from build123d import *

# Parameters (mm, degrees)
BOSS_EXTRUDE1_DEPTH = 12
SKETCH2_R           = 2.5
CUT_EXTRUDE2_DEPTH  = 1.6
SKETCH3_R           = 3
CUT_EXTRUDE3_DEPTH  = 1.6
FILLET2_R           = 1
FILLET3_R           = 1
FILLET4_R           = 1
FILLET5_R           = 1
FILLET6_R           = 1
FILLET7_R           = 1
FILLET8_R           = 1
FILLET9_R           = 1


with BuildPart() as part:
    # Sketch1 → Boss-Extrude1 (new body)
    with BuildSketch(Plane.XY):
        Polygon((-22.976789636, 1.251050745), (-7.976789636, 1.251050745), (-7.976789636, 15.251050745), (7.976789636, 15.251050745), (7.976789636, 1.251050745), (22.976789636, 1.251050745), (22.976789636, -0.348949255), (6.376789636, -0.348949255), (6.376789636, 13.651050745), (-6.376789636, 13.651050745), (-6.376789636, -0.348949255), (-22.976789636, -0.348949255), align=None)
    extrude(amount=BOSS_EXTRUDE1_DEPTH)

    # Sketch2 → Cut-Extrude2 (cut)
    with BuildSketch(Plane(origin=(0, 1.251050745, 0), x_dir=(1, 0, 0), z_dir=(0, 1, 0))):
        with Locations(Location((-16.976789636, -6, 0), (0, 0, 270))):  # turned: the seam where the file's is
            Circle(SKETCH2_R)
        with Locations(Location((16.976789636, -6, 0), (0, 0, 270))):  # turned: the seam where the file's is
            Circle(SKETCH2_R)
    extrude(amount=-CUT_EXTRUDE2_DEPTH, mode=Mode.SUBTRACT)

    # Sketch3 → Cut-Extrude3 (cut)
    with BuildSketch(Plane(origin=(0, 15.251050745, 0), x_dir=(1, 0, 0), z_dir=(0, 1, 0))):
        with Locations(Location((0, -5.812620311, 0), (0, 0, 270))):  # turned: the seam where the file's is
            Circle(SKETCH3_R)
    extrude(amount=-CUT_EXTRUDE3_DEPTH, mode=Mode.SUBTRACT)

    # Fillet2
    fillet2_edges = [part.edges().sort_by_distance(p)[0] for p in [
        (-7.976789636, 15.251050745, 6),
    ]]
    fillet(fillet2_edges, radius=FILLET2_R)

    # Fillet3
    fillet3_edges = [part.edges().sort_by_distance(p)[0] for p in [
        (7.976789636, 15.251050745, 6),
    ]]
    fillet(fillet3_edges, radius=FILLET3_R)

    # Fillet4
    fillet4_edges = [part.edges().sort_by_distance(p)[0] for p in [
        (-6.376789636, 13.651050745, 6),
    ]]
    fillet(fillet4_edges, radius=FILLET4_R)

    # Fillet5
    fillet5_edges = [part.edges().sort_by_distance(p)[0] for p in [
        (-6.376789636, -0.348949255, 6),
    ]]
    fillet(fillet5_edges, radius=FILLET5_R)

    # Fillet6
    fillet6_edges = [part.edges().sort_by_distance(p)[0] for p in [
        (6.376789636, -0.348949255, 6),
    ]]
    fillet(fillet6_edges, radius=FILLET6_R)

    # Fillet7
    fillet7_edges = [part.edges().sort_by_distance(p)[0] for p in [
        (6.376789636, 13.651050745, 6),
    ]]
    fillet(fillet7_edges, radius=FILLET7_R)

    # Fillet8
    fillet8_edges = [part.edges().sort_by_distance(p)[0] for p in [
        (-7.976789636, 1.251050745, 6),
    ]]
    fillet(fillet8_edges, radius=FILLET8_R)

    # Fillet9
    fillet9_edges = [part.edges().sort_by_distance(p)[0] for p in [
        (7.976789636, 1.251050745, 6),
    ]]
    fillet(fillet9_edges, radius=FILLET9_R)


solid = part.part
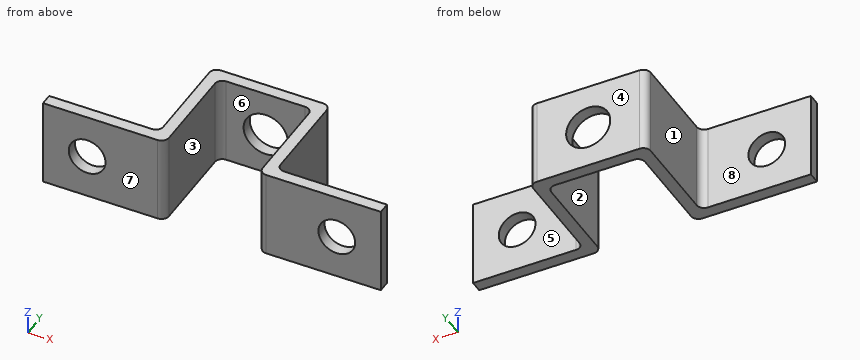
Work out the finished part from the listing and answer in its coordinate system (mm). Face numbers are marked on the shaded views. A direction names the side the tool comes from. Give positions to 0.01 mm unless a question says otherwise; leave off trailing zeros. Write each loop counter-clockwise with the first axis right and the second up, starting at its lowest first coordinate (ties: lowest second). Pieces come first, ordered by that corner, then holes.
Q1. The part is cut by section C-C on z = 1.5. Give the vertices of the cut face in (x, y).
Answer:
outline: (-22.98, -0.35) - (-7.38, -0.35) arc R1 ccw to (-6.38, 0.65) - (-6.38, 12.65) arc R1 cw to (-5.38, 13.65) - (5.38, 13.65) arc R1 cw to (6.38, 12.65) - (6.38, 0.65) arc R1 ccw to (7.38, -0.35) - (22.98, -0.35) - (22.98, 1.25) - (8.98, 1.25) arc R1 cw to (7.98, 2.25) - (7.98, 14.25) arc R1 ccw to (6.98, 15.25) - (-6.98, 15.25) arc R1 ccw to (-7.98, 14.25) - (-7.98, 2.25) arc R1 cw to (-8.98, 1.25) - (-22.98, 1.25) - close
Q2. Given pin 1 (6 mm diameter, centred on x = 17.5, z = 7.5, fed in from +Y); pin 2 (6 mm diameter, centred on y = 8, z = 3.5, fed in from -X); pin 3 (2 mm diameter, centred on y = 7, z = 7.5, fed in from +X), each flat-ended and moving along its own axis, determine where each tip first touches the part or whether it passes through.
Answer:
pin 1: stops at y = 1.25
pin 2: stops at x = -7.98
pin 3: stops at x = 7.98
Q3. The part is cut by section A-A on x = 0. Give the vertices of the cut face in (y, z).
Answer:
outline: (13.65, 0) - (15.25, 0) - (15.25, 2.81) - (13.65, 2.81) - close; (13.65, 8.81) - (15.25, 8.81) - (15.25, 12) - (13.65, 12) - close
Q4. Straight lines are drawn through the part: L1, parallel to X at y = 0.6, z = 6; L2, parallel to X at y = 11.75, z = 2; L3, parallel to X at y = 0.5, z = 5. For each, find the intervals that lie inside material, in ascending order.
Answer:
L1: x = -22.98 to -19.48, -14.48 to -6.38, 6.38 to 14.48, 19.48 to 22.98
L2: x = -7.98 to -6.38, 6.38 to 7.98
L3: x = -22.98 to -19.27, -14.69 to -6.39, 6.39 to 14.69, 19.27 to 22.98
Q5. For a pull along X with two mould halves and no side action, classify the marked faces 1, 2, 3 and 4 as released by +X, released by -X, zero draft, split by the parting line, or undercut.
Answer:
face 1: released by -X
face 2: undercut
face 3: undercut
face 4: zero draft
Q6. The part is cut by section D-D on z = 5. State how many separate pieces and enclosed holes the cut face has, and give its area (3 significant figures).
Answer:
separate pieces: 4
enclosed holes: 0
area: 94.4 mm2
Q7. The part is cut by section B-B on y = 10.25. Give the vertices of the cut face in (x, z).
Answer:
outline: (-7.98, 0) - (-6.38, 0) - (-6.38, 12) - (-7.98, 12) - close; (6.38, 0) - (7.98, 0) - (7.98, 12) - (6.38, 12) - close
Q8. A tool of negligible diameter and unlimited length cuts with its end or side. For the marked faces 5, 6, 7 and 8, from which of +Z, -Z, +X, -X, +Y, -Y can it reach the whole face along a straight path? Write none if from no direction.
Answer:
face 5: +Z, -Z, +X, +Y
face 6: +Z, -Z, -Y
face 7: +Z, -Z, +X, -X, -Y
face 8: +Z, -Z, -X, +Y
